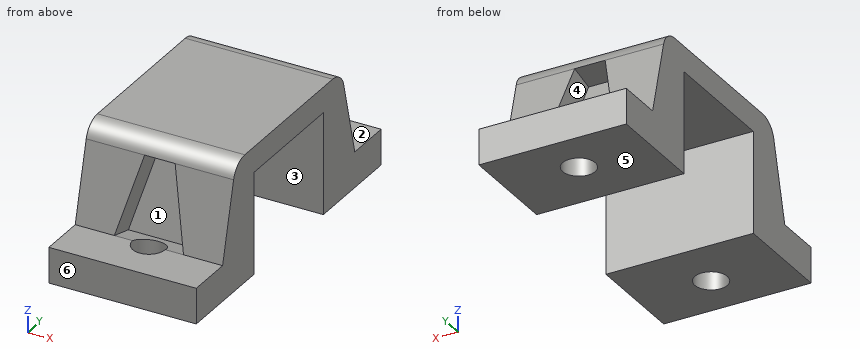
Autodesk Inventor part; units mm, degrees
ref_plane "YZ Plane" through (0, 0, 0) normal (1, 0, 0) x (0, 1, 0)
ref_plane "XZ Plane" through (0, 0, 0) normal (0, 1, 0) x (-1, 0, 0)
ref_plane "XY Plane" through (0, 0, 0) normal (0, 0, 1) x (1, 0, 0)
sketch "Sketch1" plane through (0, 0, 0) normal (1, 0, 0) x (0, 1, 0)
  line L0 (-6, -5) -> (0, -5) construction
  line L1 (6, -5) -> (6, 5)
  line L2 (6, 5) -> (-6, 5)
  line L3 (-6, 5) -> (-6, -5)
  line L4 (-6, -5) -> (6, 5) construction
  line L5 (6, -5) -> (-6, 5) construction
  line L6 (-7.5995, 7.5) -> (7.5995, 7.5)
  line L7 (9.1552, -7.5) -> (-9.1552, 7.5) construction
  line L8 (-9.1552, -7.5) -> (9.1552, 7.5) construction
  line L9 (9.1552, -7.5) -> (9, -7.5)
  line L10 (-9, -7.5) -> (-9.1552, -7.5)
  line L11 (-6, -5) -> (-16, -5)
  line L12 (-16, -5) -> (-16, -1.5)
  line L13 (-16, -1.5) -> (-11.44, -1.5)
  line L14 (-11.44, -1.5) -> (-9.538, 5.9921)
  line L15 (0, 0) -> (0, 13.1521) construction
  line L16 (9.1552, -7.5) -> (-9.1552, 7.5) construction
  line L17 (9, -7.5) -> (9.1552, -7.5)
  line L18 (6, -5) -> (16, -5)
  line L19 (16, -5) -> (16, -1.5)
  line L20 (16, -1.5) -> (11.44, -1.5)
  line L21 (11.44, -1.5) -> (9.538, 5.9921)
  arc A0 (-7.5995, 7.5) -> (-9.538, 5.9921) centre (-7.5995, 5.5) ccw
  arc A1 (9.538, 5.9921) -> (7.5995, 7.5) centre (7.5995, 5.5) ccw
  dimension "d0" = 12
  dimension "d1" = 10
  dimension "d2" = 2.5
  dimension "d3" = 10
  dimension "d4" = 3.5
  dimension "d5" = 4.56
  dimension "d6" = 2
extrude "Extrusion1" add sketch "Sketch1" along normal blind 14.5
sketch "Sketch2" plane through (0, 9.538, 5.9921) normal (0, 0.9693, 0.2461) x (1, 0, 0)
  line L0 (0, 7.7298) -> (14.5, 7.7298)
  line L1 (7.25, 7.7298) -> (15.5846, 7.7298) construction
  line L2 (7.25, 7.7298) -> (7.25, 0) construction
  line L3 (7.25, 0) -> (8.75, 0)
  line L4 (0, 0) -> (14.5, 0)
  line L5 (7.25, 0) -> (5.75, 0)
  line L6 (7.25, 7.7298) -> (10.65, 7.7298)
  line L7 (7.25, 7.7298) -> (3.85, 7.7298)
  line L8 (3.85, 7.7298) -> (5.75, 0)
  line L9 (10.65, 7.7298) -> (8.75, 0)
  point P0 (0, 3.461)
  point P1 (10.65, 7.7298)
  dimension "d13" = 1.5
  dimension "d14" = 1.5
  dimension "d15" = 3.4
  dimension "d16" = 3.4
extrude "Extrusion2" cut sketch "Sketch2" against normal blind 2.5
sketch "Sketch3" plane through (0, 11.44, -1.5) normal (0, 0, 1) x (1, 0, 0)
  line L0 (0, 4.56) -> (14.5, 4.56) construction
  line L1 (14.5, 4.56) -> (7.25, 0) construction
  line L2 (3.85, 0) -> (10.65, 0) construction
  line L3 (0, 4.56) -> (7.25, 0) construction
  circle A0 centre (7.25, 0) radius 1.6
  point P0 (0, -11.44)
  dimension "d19" = 3.2
extrude "Extrusion3" cut sketch "Sketch3" against normal blind 4
sketch "Sketch4" plane through (0, -11.44, -1.5) normal (0, -0.9693, 0.2461) x (1, 0, 0)
  line L0 (0, 0) -> (14.5, 0)
  line L1 (7.25, 0) -> (10.65, 0) construction
  line L2 (7.25, 0) -> (7.25, 7.6387) construction
  line L3 (7.25, 0) -> (3.85, 0) construction
  line L4 (7.25, 0) -> (10.65, 0)
  line L5 (7.25, 0) -> (3.85, 0)
  line L6 (7.25, 7.3642) -> (7.25, 7.7298) construction
  line L7 (0, 7.7298) -> (14.5, 7.7298) construction
  line L8 (7.25, 7.7298) -> (5.75, 7.7298)
  line L9 (7.25, 7.7298) -> (8.75, 7.7298)
  line L10 (3.85, 0) -> (5.75, 7.7298)
  line L11 (10.65, 0) -> (8.75, 7.7298)
  point P0 (0, 4.2688)
  dimension "d22" = 3.4
  dimension "d23" = 3.4
  dimension "d25" = 1.5
  dimension "d26" = 1.5
extrude "Extrusion4" cut sketch "Sketch4" against normal blind 2.5
sketch "Sketch5" plane through (0, -16, -1.5) normal (0, 0, 1) x (1, 0, 0)
  line L0 (0, 4.56) -> (0, 0) construction
  line L1 (0, 0) -> (7.25, 4.56) construction
  line L2 (3.85, 4.56) -> (10.65, 4.56) construction
  line L3 (14.5, 4.56) -> (14.5, 0) construction
  line L4 (14.5, 0) -> (7.25, 4.56) construction
  circle A0 centre (7.25, 4.56) radius 1.6
  point P0 (0, 16)
  dimension "d29" = 3.2
extrude "Extrusion5" cut sketch "Sketch5" against normal blind 4
properties part number "soporte_motor"
Build history of the part. All positions in model axes, mm. Face numbers are marked on the shaded views. A direction names the side the tool comes from. Round coordinates to 2 decimals unless told otherwise and drop trailing zeros. Write each loop counter-clockwise with the first axis right and the second up, starting at its lowest first coordinate (ties: lowest second). Pieces come first, ordered by that corner, then holes. Notation, with made-up numbers: (23, 56) -> (62, 56) arc R33 cw to (62, 89) -> close; hole circle Ø3 at (11, -14). An arc over 180 degrees is marked (long way). Put each result on its own line as item: value.
Item 1: Slice it at B-B, the plane x = 7.25. Give the cut face in (y, z).
Here are the results:
outline: (-16, -5) -> (-13.04, -5) -> (-13.04, -1.5) -> (-16, -1.5) -> close; (-9.84, -5) -> (-6, -5) -> (-6, 5) -> (6, 5) -> (6, -5) -> (9.84, -5) -> (9.84, -1.91) -> (9.02, -2.12) -> (7.11, 5.38) -> (9.54, 5.99) arc R2 ccw to (7.6, 7.5) -> (-7.6, 7.5) arc R2 ccw to (-9.54, 5.99) -> (-7.11, 5.38) -> (-9.01, -2.12) -> (-9.84, -1.91) -> close; (13.04, -5) -> (16, -5) -> (16, -1.5) -> (13.04, -1.5) -> close
Item 2: Slice it at C-C, the plane z = 0. Give the cut face in (x, y).
Here are the results:
outline: (0, -11.06) -> (4.23, -11.06) -> (4.39, -8.48) -> (10.11, -8.48) -> (10.27, -11.06) -> (14.5, -11.06) -> (14.5, -6) -> (0, -6) -> close; (0, 6) -> (14.5, 6) -> (14.5, 11.06) -> (10.27, 11.06) -> (10.11, 8.48) -> (4.39, 8.48) -> (4.23, 11.06) -> (0, 11.06) -> close
Item 3: Slice it at A-A, the plane z = -3. Give the cut face in (x, y), plus the area to 3 significant figures.
Here are the results:
outline: (0, -16) -> (14.5, -16) -> (14.5, -6) -> (0, -6) -> close; (0, 6) -> (14.5, 6) -> (14.5, 16) -> (0, 16) -> close; hole circle Ø3.2 at (7.25, -11.44); hole circle Ø3.2 at (7.25, 11.44)
area: 274 mm^2
Item 4: Two-plate mould, pull along Z, no slides. Class the marked faces 4, 5 and 6: pulls with the +Z half, pulls with the -Z half, needs draft (parallel to the pull), parting line crosses it, or undercut.
Here are the results:
face 4: undercut
face 5: pulls with the -Z half
face 6: needs draft
Item 5: Flat gauge pins, fed straight in: P1, Ø5, axis at x = 5.5, z = 0, coming from the -Y side; P2, Ø1.4, axis at x = 8.5, y = -13.5, coming from the +Z side; P3, Ø3.5, axis at x = 4, y = -2.5, coming from the -Z side; P4, Ø2, axis at x = 11, z = 3.5, coming from the -Y side. Where does each tip first touch, or does it go through?
Here are the results:
P1: stops at y = -16
P2: stops at z = -1.5
P3: stops at z = 5
P4: stops at y = -10.42
Item 6: Tool access for the marked faces 1, 2 and 3: list every direction of +Z, -Z, +X, -X, +Y, -Y with a clear straight run to the whole face (end or side of a thin tool).
Here are the results:
face 1: none
face 2: +Z, +X, -X, +Y
face 3: -Z, +X, -X
Item 7: Wall check: probe 1 along Y at (x, z) = (7.25, -4.2); probe 2 along X at (y, z) = (-11.44, -3.65); probe 3 along X at (y, z) = (12, -4). Give the ranges that are in metal, low to high. Write a range as from..to.
Here are the results:
probe 1: y = -16..-13.04, -9.84..-6, 6..9.84, 13.04..16
probe 2: x = 0..5.65, 8.85..14.5
probe 3: x = 0..5.75, 8.75..14.5
Item 8: Slice it at D-D, the plane y = 8.5. Give the cut face in (x, z).
Here are the results:
outline: (0, -5) -> (14.5, -5) -> (14.5, 7.29) -> (0, 7.29) -> close; hole (4.36, -0.09) -> (10.14, -0.09) -> (8.75, 5.73) -> (5.75, 5.73) -> close
